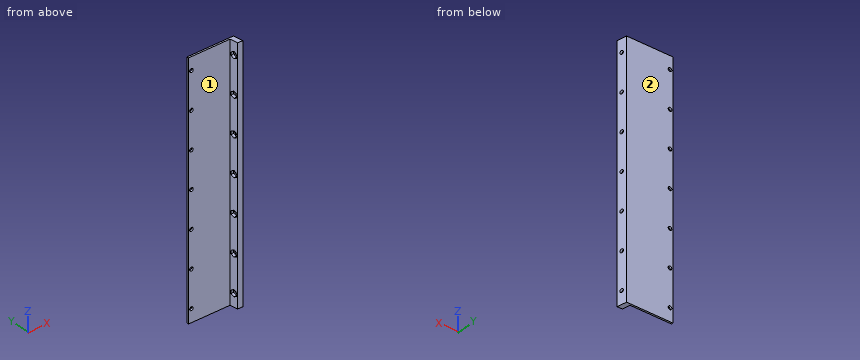
from build123d import *

# Parameters (mm, degrees)
BOSS_EXTRUDE1_DEPTH = 171
SKETCH2_R           = 1.25
CUT_EXTRUDE1_DEPTH  = 50
SKETCH3_R           = 1.25
CUT_EXTRUDE2_DEPTH  = 50
CUT_EXTRUDE3_DEPTH  = 2
LPATTERN1_COUNT     = 7
LPATTERN1_PITCH     = 25.5


with BuildPart() as part:
    # Sketch1 → Boss-Extrude1 (new body)
    with BuildSketch(Plane.XY):
        Polygon((0, 0), (32.09, 0), (33.178500502, -6.66165645), (29.624787969, -6.61699683), (28.739662203, -1.2), (0, -1.2), align=None)
    extrude(amount=BOSS_EXTRUDE1_DEPTH)

    # Sketch2 → Cut-Extrude1 (cut)
    with BuildSketch(Plane(origin=(0, 0, 0), x_dir=(1, 0, 0), z_dir=(0, 1, 0))):
        with Locations(Location((2, -9, 0), (0, 0, 270))):
            Circle(SKETCH2_R)
    cut_extrude1 = extrude(amount=-CUT_EXTRUDE1_DEPTH, mode=Mode.SUBTRACT)

    # Sketch3 → Cut-Extrude2 (cut)
    with BuildSketch(Plane(origin=(31.255513263, 5.107084422, 0), x_dir=(0, 0, -1), z_dir=(0.9869120666582158, 0.16125933363501674, 0))):
        with Locations(Location((-9, -8.674812016, 0), (0, 0, 90))):
            Circle(SKETCH3_R)
    cut_extrude2 = extrude(amount=-CUT_EXTRUDE2_DEPTH, mode=Mode.SUBTRACT)

    # Sketch4 → Cut-Extrude3 (cut)
    with BuildSketch(Plane(origin=(27.801321029, 4.542676754, 0), x_dir=(0, 0, 1), z_dir=(-0.9869120666582157, -0.1612593336350174, 0))):
        Polygon((7.816431948, -6.624812016), (6.632863896, -8.674812016), (7.816431948, -10.724812016), (10.183568052, -10.724812016), (11.367136104, -8.674812016), (10.183568052, -6.624812016), align=None)
    cut_extrude3 = extrude(amount=-CUT_EXTRUDE3_DEPTH, mode=Mode.SUBTRACT)

    # LPattern1: Cut-Extrude1, Cut-Extrude2, Cut-Extrude3 ×7
    with Locations(*[(0, 0, i * LPATTERN1_PITCH) for i in range(1, LPATTERN1_COUNT)]):
        add(cut_extrude1, mode=Mode.SUBTRACT)
        add(cut_extrude2, mode=Mode.SUBTRACT)
        add(cut_extrude3, mode=Mode.SUBTRACT)


solid = part.part
Here's how the part is built. I have some questions about the finished solid (model axes, mm). Face numbers are marked on the shaded views. A direction names the side the tool comes from. Round coordinates to 2 decimals unless told otherwise and drop trailing zeros. Write each loop counter-clockwise with the first axis right and the second up, starting at its lowest first coordinate (ties: lowest second). Pieces come first, ordered by that corner, then holes.
1. Suppose I cut it at B-B (x = 7). List the corners of the cut face in (y, z) for me, and give its area (3 significant figures).
2. I need wall thicknesses on L1, parallel to X at y = -0.3, z = 34.5; L2, parallel to Y at x = 14.5, z = 101; L3, parallel to X at y = -0.6, z = 85.5. Which ranges of each line are inside material? Lowest first, please.
3. Will these pins go through, and if not, where does the flat tip stop? pin 1 Ø3 at (x, z) = (2, 162) entering from +Y; pin 2 Ø3 at (x, z) = (2, 60) entering from -Y; pin 3 Ø1.5 at (x, z) = (2, 34.5) entering from +Y.
4. Suppose I cut it at A-A (z = 21). List the corners of the cut face in (x, y) for me.
5. For the marked faces 1 and 2, which set-ups out of +Z, -Z, +X, -X, +Y, -Y let a thin tool reach every point of the face, with its end or its side?
Answer sheet:
1. outline: (-1.2, 0) - (0, 0) - (0, 171) - (-1.2, 171) - close
1. area: 205 mm2
2. L1: x = 0 to 0.75, 3.25 to 32.14
2. L2: y = -1.2 to 0
2. L3: x = 0 to 0.75, 3.25 to 32.19
3. pin 1: stops at y = 0
3. pin 2: stops at y = -1.2
3. pin 3: passes through
4. outline: (0, -1.2) - (28.74, -1.2) - (29.62, -6.62) - (33.18, -6.66) - (32.09, 0) - (0, 0) - close
5. face 1: +Z, -Z, -X, -Y
5. face 2: +Z, -Z, +X, -X, +Y
